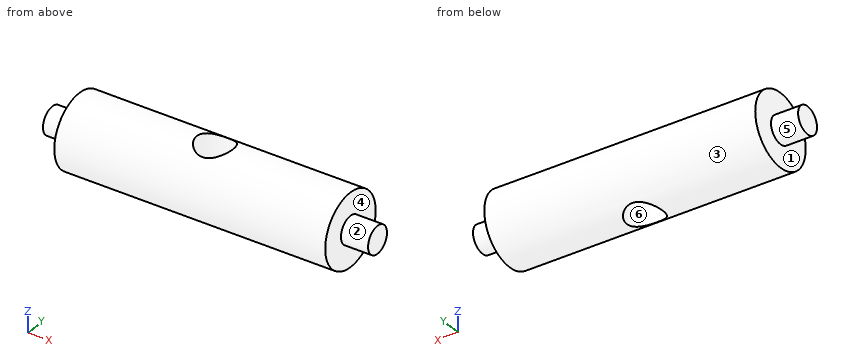
```python
from build123d import *

# Parameters (mm, degrees)
F2_R     = 2
F3_DEPTH = 5


with BuildPart() as f1:
    # F0 (on Top) → F1 (revolve)
    with BuildSketch(Plane.XY):
        Polygon((-18, 1.5), (-18, 0), (18, 0), (18, 1.5), (15, 1.5), (15, 4), (-15, 4), (-15, 1.5), align=None)
    revolve(axis=Axis((0, 0, 0), (-1, 0, 0)))

    # F2 (on Top) → F3 (cut, symmetric)
    with BuildSketch(Plane.XY):
        Circle(F2_R)
    extrude(amount=F3_DEPTH, both=True, mode=Mode.SUBTRACT)


solid = f1.part
```
Work out the finished part from the listing and answer in its coordinate system (mm). Face numbers are marked on the shaded views. A direction names the side the tool comes from. Give positions to 0.01 mm unless a question says otherwise; leave off trailing zeros. Write each loop counter-clockwise with the first axis right and the second up, starting at its lowest first coordinate (ties: lowest second). Pieces come first, ordered by that corner, then holes.
(1) The mould has two halves that part along X. Classify the marked faces 4, 5 and 6: pulls with the +X half, pulls with the -X half, needs draft (parallel to the pull), parting line crosses it, or undercut.
Final values:
face 4: pulls with the +X half
face 5: needs draft
face 6: undercut
(2) Which of the six approach directions +Z, -Z, +X, -X, +Y, -Y give full straight-line access (tool end or side, diameter ignored) to the marked faces 1, 2 and 3?
Final values:
face 1: -X
face 2: +X
face 3: +X, -X
(3) The part is cut by section B-B on z = -0.5. Write down the section's boundary in (x, y), plus the area to 3 significant figures.
Final values:
outline: (-18, -1.41) - (-15, -1.41) - (-15, -3.97) - (15, -3.97) - (15, -1.41) - (18, -1.41) - (18, 1.41) - (15, 1.41) - (15, 3.97) - (-15, 3.97) - (-15, 1.41) - (-18, 1.41) - close; hole circle Ø4 at (0, 0)
area: 243 mm2
(4) The part is cut by section A-A on y = 0. Write down the section's boundary in (x, z).
Final values:
outline: (-18, -1.5) - (-15, -1.5) - (-15, -4) - (-2, -4) - (-2, 4) - (-15, 4) - (-15, 1.5) - (-18, 1.5) - close; (2, -4) - (15, -4) - (15, -1.5) - (18, -1.5) - (18, 1.5) - (15, 1.5) - (15, 4) - (2, 4) - close
(5) Straight lines are drawn through the part: line 1 (Y direction, x = 0, z = -0.25); line 2 (X direction, y = 0, z = 1); line 3 (X direction, y = -2.75, z = -1.75). For each, find the intervals that lie inside material, in ascending order.
Final values:
line 1: y = -3.99 to -2, 2 to 3.99
line 2: x = -18 to -2, 2 to 18
line 3: x = -15 to 15
(6) The part is cut by section D-D on x = -13. Write down the section's boundary in (y, z).
Final values:
outline: circle Ø8 at (0, 0)
(7) Flat-ended cylindrical pins translate along their axes: pin 1 Ø1.5 at (y, z) = (-3, 2) entering from -X; pin 2 Ø1.5 at (x, z) = (0.5, 2) entering from +Y. Find the tip coordinate at first contact, or state that the pin passes through.
Final values:
pin 1: stops at x = -15
pin 2: stops at y = 3.8
(8) The part is cut by section C-C on x = 0. Write down the section's boundary in (y, z), plus the area to 3 significant figures.
Final values:
outline: (-2, -3.46) - (-2, 3.46) arc R4 ccw to start; (2, -3.46) arc R4 ccw to (2, 3.46) - close
area: 19.7 mm2
